Can you work these out from the model? Positions are in its coordinate system, mm. Face numbers are marked on the shaded views. A direction names the side the tool comes from. Coordinates: 2 decimals unless noted, no trailing zeros. Order: outer loops, then holes, each group sorted by start corner. A loop starts at its lowest first (then second) coordinate and runs counter-clockwise, first axis right, second up. Notation, with made-up numbers: (87.25, 37) - (130.25, 37) arc R11 cw to (130.25, 41) - close; hole circle Ø7 at (-16.75, 58). An arc over 180 degrees is marked (long way). Return JSON: item names as keys, results as strings. Group by question number.
1) For pin 1 Ø11 at (x, y) = (-22.86, 12.7) entering from -Z; pin 2 Ø2 at (x, y) = (9.5, 26) entering from -Z; pin 3 Ø1.5 at (y, z) = (45.5, -92.5) entering from -X, each with a flat end and sliding along its axis, tell me the tip position at first contact or that it passes through.
2) Which directions (+Z, -Z, +X, -X, +Y, -Y) give clear straight access to the entire face, cutting with the end or side of a thin tool? Please do the marked faces 1 and 2.
3) Imagine slicing it at A-A (y = 12.7). Write out the boundary of the cut face in (x, z), and give its area (3 significant figures).
4) Imagine slicing it at B-B (z = -40). Write out the boundary of the cut face in (x, y), and give its area (3 significant figures).
5) Imagine slicing it at D-D (x = -22.86). Write out the boundary of the cut face in (y, z), and give its area (3 significant figures).
6) If we mould it in two halves opening along Z, with no side actions, what happens to the marked faces 3, 4 and 5? For each: pulls with the +Z half, pulls with the -Z half, needs draft (parallel to the pull), parting line crosses it, or undercut.
7) If I drill on line 1 along X through (y, z) = (47.5, -41); line 2 along Y through (x, z) = (-22.86, -1.75); line 3 along X through (y, z) = (12, -1), over which ranges is the centre line in solid material (lowest first)?
8) Imagine slicing it at C-C (y = 39). Write out the boundary of the cut face in (x, z), and give its area (3 significant figures).
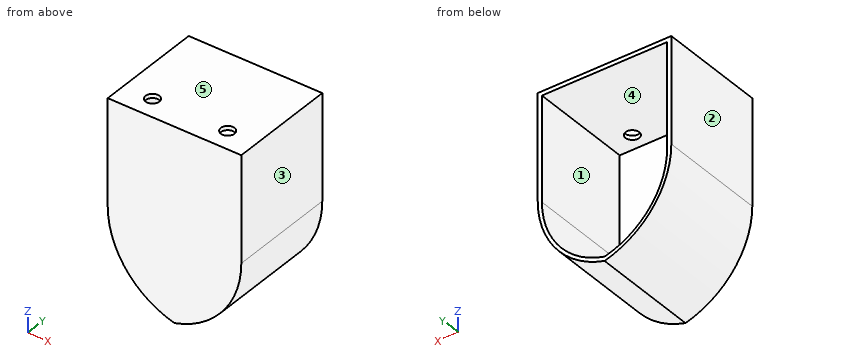
```python
from build123d import *

# Parameters (mm, degrees)
BOSS_EXTRUDE1_DEPTH = 66.04
THICKEN1_T2         = 2.54
SKETCH3_R           = 4.191
CUT_EXTRUDE1_DEPTH  = 2.54


with BuildPart() as part:
    # Sketch1 → Boss-Extrude1 (new body)
    with BuildSketch(Plane(origin=(0, 0, 0), x_dir=(1, 0, 0), z_dir=(0, 1, 0))):
        with BuildLine():
            Line((40.64, 0), (-40.64, 0))
            Line((-40.64, 0), (-40.64, 64.32775415))
            ThreePointArc((-40.64, 64.32775415), (-29.293308759, 97.528452803), (0, 116.84))
            ThreePointArc((0, 116.84), (29.293308759, 97.528452803), (40.64, 64.32775415))
            Line((40.64, 64.32775415), (40.64, 0))
        make_face()
        with BuildLine():
            Line((-38.1, 2.54), (38.1, 2.54))
            Line((38.1, 2.54), (38.1, 65.938950101))
            ThreePointArc((38.1, 65.938950101), (27.430794734, 96.722067013), (0, 114.3))
            ThreePointArc((0, 114.3), (-27.430794734, 96.722067013), (-38.1, 65.938950101))
            Line((-38.1, 65.938950101), (-38.1, 2.54))
        make_face(mode=Mode.SUBTRACT)
    extrude(amount=BOSS_EXTRUDE1_DEPTH)

    # Sketch2 → Surface-Plane1: a flat surface bounded by the sketch
    with BuildSketch(Plane.XZ, mode=Mode.PRIVATE) as surface_plane1_1_region:
        with BuildLine():
            Line((-40.64, 0), (40.64, 0))
            Line((40.64, 0), (40.64, -64.32775415))
            ThreePointArc((40.64, -64.32775415), (29.293308759, -97.528452803), (0, -116.84))
            ThreePointArc((0, -116.84), (-29.293308759, -97.528452803), (-40.64, -64.32775415))
            Line((-40.64, -64.32775415), (-40.64, 0))
        make_face()
    surface_plane1_1 = surface_plane1_1_region.sketch.faces()[0]
    add(Solid.thicken(surface_plane1_1, -THICKEN1_T2))

    # Sketch3 → Cut-Extrude1 (cut)
    with BuildSketch(Plane.XY):
        with Locations((22.86, 12.7)):
            Circle(SKETCH3_R)
        with Locations((-22.86, 12.7)):
            Circle(SKETCH3_R)
    extrude(amount=-CUT_EXTRUDE1_DEPTH, mode=Mode.SUBTRACT)


solid = part.part
```
Calculated:
{
 "1": {"pin 1": "z = -108.87", "pin 2": "z = -113.87", "pin 3": "x = -33.2"},
 "2": {"face 1": "+Y", "face 2": "+Z, -Z, -X, +Y, -Y"},
 "3": {"outline": "(-40.64, -64.33) arc R54.25 ccw to (0, -116.84) arc R54.25 ccw to (40.64, -64.33) - (40.64, 0) - (27.05, 0) - (27.05, -2.54) - (38.1, -2.54) - (38.1, -65.94) arc R49.74 cw to (0, -114.3) arc R49.74 cw to (-38.1, -65.94) - (-38.1, -2.54) - (-27.05, -2.54) - (-27.05, 0) - (-40.64, 0) - close; (-18.67, -2.54) - (18.67, -2.54) - (18.67, 0) - (-18.67, 0) - close", "area": "778 mm2"},
 "4": {"outline": "(-40.64, 0) - (40.64, 0) - (40.64, 66.04) - (38.1, 66.04) - (38.1, 2.54) - (-38.1, 2.54) - (-38.1, 66.04) - (-40.64, 66.04) - close", "area": "529 mm2"},
 "5": {"outline": "(0, -104.49) - (66.04, -104.49) - (66.04, -101.77) - (2.54, -101.77) - (2.54, -2.54) - (8.51, -2.54) - (8.51, 0) - (0, 0) - close; (16.89, -2.54) - (66.04, -2.54) - (66.04, 0) - (16.89, 0) - close", "area": "578 mm2"},
 "6": {"face 3": "needs draft", "face 4": "undercut", "face 5": "pulls with the +Z half"},
 "7": {"line 1": "-40.64 to -38.1, 38.1 to 40.64", "line 2": "0 to 8.51, 16.89 to 66.04", "line 3": "-40.64 to -26.99, -18.73 to 18.73, 26.99 to 40.64"},
 "8": {"outline": "(-40.64, -64.33) arc R54.25 ccw to (0, -116.84) arc R54.25 ccw to (40.64, -64.33) - (40.64, 0) - (-40.64, 0) - close; hole (-38.1, -65.94) arc R49.74 ccw to (0, -114.3) arc R49.74 ccw to (38.1, -65.94) - (38.1, -2.54) - (-38.1, -2.54) - close", "area": "820 mm2"}
}
